from build123d import *

# Parameters (mm, degrees)
SKETCH1_W           = 35
SKETCH1_H           = 30
SKETCH1_R           = 2.75
SKETCH1_R_2         = 1
BOSS_EXTRUDE1_DEPTH = 1.5
SKETCH2_W           = 35
SKETCH2_H           = 30
BOSS_EXTRUDE2_DEPTH = 6.5
SKETCH3_R           = 1.5
CUT_EXTRUDE1_DEPTH  = 9
FILLET1_R           = 2


with BuildPart() as part:
    # Sketch1 → Boss-Extrude1 (new body)
    with BuildSketch(Plane(origin=(0, 0, 0), x_dir=(1, 0, 0), z_dir=(0, 1, 0))):
        Rectangle(SKETCH1_W, SKETCH1_H)
        with Locations((-6.32455, -4)):
            Circle(SKETCH1_R, mode=Mode.SUBTRACT)
        with Locations((0, 5)):
            Circle(SKETCH1_R_2, mode=Mode.SUBTRACT)
    extrude(amount=BOSS_EXTRUDE1_DEPTH)

    # Sketch2 → Boss-Extrude2 (add)
    with BuildSketch(Plane(origin=(0, 1.5, 0), x_dir=(1, 0, 0), z_dir=(0, 1, 0))):
        Rectangle(SKETCH2_W, SKETCH2_H)
        Polygon((-10.5, 13), (10.5, 13), (10.5, 8), (15.5, 8), (15.5, -8), (10.5, -8), (10.5, -13), (-10.5, -13), (-10.5, -8), (-15.5, -8), (-15.5, 8), (-10.5, 8), align=None, mode=Mode.SUBTRACT)
    extrude(amount=BOSS_EXTRUDE2_DEPTH)

    # Sketch3 → Cut-Extrude1 (cut, through all)
    with BuildSketch(Plane(origin=(0, 8, 0), x_dir=(1, 0, 0), z_dir=(0, 1, 0))):
        with Locations((-14, 11.5)):
            Circle(SKETCH3_R)
        with Locations((-14, -11.5)):
            Circle(SKETCH3_R)
        with Locations((14, -11.5)):
            Circle(SKETCH3_R)
        with Locations((14, 11.5)):
            Circle(SKETCH3_R)
    extrude(amount=-CUT_EXTRUDE1_DEPTH, mode=Mode.SUBTRACT)

    # Fillet1
    fillet1_edges = [part.edges().sort_by_distance(p)[0] for p in [
        (-10.5, 4.75, -8),
        (-10.5, 4.75, 8),
        (10.5, 4.75, 8),
        (10.5, 4.75, -8),
        (17.5, 4, 15),
        (-17.5, 4, 15),
        (-17.5, 4, -15),
        (17.5, 4, -15),
    ]]
    fillet(fillet1_edges, radius=FILLET1_R)


solid = part.part
Verification items for the finished model (mm, model axes). A direction names the side the tool comes from. Give positions to 0.01 mm unless a question says otherwise; leave off trailing zeros. Loops run counter-clockwise (first coordinate to the right, second up) from the corner with the lowest first, then second, coordinate; pieces in that order, holes last.
1) Draft check along X on faces 3 (the flat face through (0, 4, 15)), 4 (the flat face through (-14, 5, -8)), 5 (the cylindrical face through (16.9, 3.94, -14.43)). Enter one of: pulls with the +X half, pulls with the -X half, needs draft (parallel to the pull), parting line crosses it, or undercut.
2) Set-up check for faces 1 (the flat face through (0, 1.5, 0)), 2 (the cylindrical face through (-15.5, 4.06, 11.43)): record each of +Z, -Z, +X, -X, +Y, -Y from which the full face is reachable in a straight line by a thin tool's end or side.
3) Sectioned sample at B-B, the plane x = 0. Enter the section's corners in (y, z).
4) Thickness scan on line 1 along X through (y, z) = (5.75, 11.5); line 2 along Z through (x, y) = (14, 3); line 3 along Z through (x, y) = (-4, 7.25). Record the ranges inside material, lowest first.
5) Sectioned sample at D-D, the plane y = 2.25. Enter the section's corners in (x, z).
6) Sectioned sample at C-C, the plane z = 4. Enter the section's corners in (x, y).
7) Sectioned sample at A-A, the plane x = -14. Enter the section's corners in (y, z).
8) Depth check by flat-ended pin: pin 1 Ø1 at (x, z) = (11, 8.5) entering from -Y; pin 2 Ø6.5 at (x, z) = (-6.32, 4) entering from +Y. Enter the tip coordinate at first touch or a pass-through.
Answers:
1. face 3: needs draft
1. face 4: undercut
1. face 5: pulls with the +X half
2. face 1: +Y
2. face 2: +Y, -Y
3. outline: (0, -15) - (8, -15) - (8, -13) - (1.5, -13) - (1.5, -6) - (0, -6) - close; (0, -4) - (1.5, -4) - (1.5, 13) - (8, 13) - (8, 15) - (0, 15) - close
4. line 1: x = -17.5 to -15.5, -12.5 to -10.5, 10.5 to 12.5, 15.5 to 17.5
4. line 2: z = -15 to -13, -10 to -8, 8 to 10, 13 to 15
4. line 3: z = -15 to -13, 13 to 15
5. outline: (-17.5, -13) arc R2 ccw to (-15.5, -15) - (15.5, -15) arc R2 ccw to (17.5, -13) - (17.5, 13) arc R2 ccw to (15.5, 15) - (-15.5, 15) arc R2 ccw to (-17.5, 13) - close; hole circle Ø3 at (-14, -11.5); hole (-15.5, -8) - (-12.5, -8) arc R2 cw to (-10.5, -10) - (-10.5, -13) - (10.5, -13) - (10.5, -10) arc R2 cw to (12.5, -8) - (15.5, -8) - (15.5, 8) - (12.5, 8) arc R2 cw to (10.5, 10) - (10.5, 13) - (-10.5, 13) - (-10.5, 10) arc R2 cw to (-12.5, 8) - (-15.5, 8) - close; hole circle Ø3 at (-14, 11.5); hole circle Ø3 at (14, -11.5); hole circle Ø3 at (14, 11.5)
6. outline: (-17.5, 0) - (-9.07, 0) - (-9.07, 1.5) - (-15.5, 1.5) - (-15.5, 8) - (-17.5, 8) - close; (-3.57, 0) - (17.5, 0) - (17.5, 8) - (15.5, 8) - (15.5, 1.5) - (-3.57, 1.5) - close
7. outline: (0, -15) - (8, -15) - (8, -13) - (0, -13) - close; (0, -10) - (8, -10) - (8, -8) - (1.5, -8) - (1.5, 8) - (8, 8) - (8, 10) - (0, 10) - close; (0, 13) - (8, 13) - (8, 15) - (0, 15) - close
8. pin 1: stops at y = 0
8. pin 2: stops at y = 1.5
